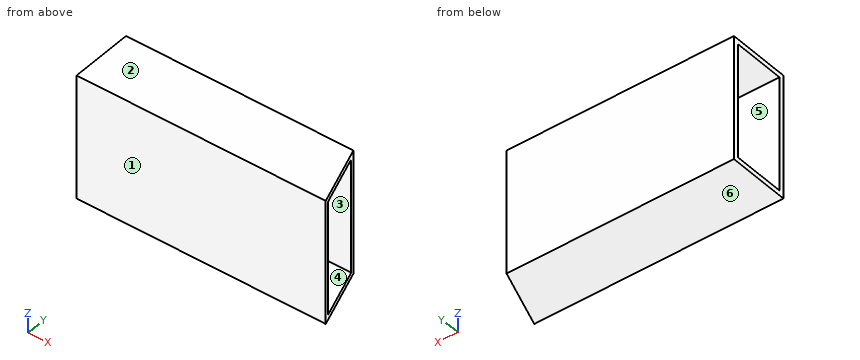
```python
from build123d import *

# Parameters (mm, degrees)
DODANIE_WYCI_GNI_CIE1_DEPTH = 100
SZKIC2_W                    = 92
SZKIC2_H                    = 42
WYTNIJ_WYCI_GNI_CIE1_DEPTH  = 200


with BuildPart() as part:
    # Szkic1 → Dodanie-wyciągnięcie1 (new body)
    with BuildSketch(Plane.XY):
        Polygon((0, 0), (200, 0), (182.5, 50), (0, 50), align=None)
    extrude(amount=DODANIE_WYCI_GNI_CIE1_DEPTH)

    # Szkic2 → Wytnij-wyciągnięcie1 (cut)
    with BuildSketch(Plane.ZY):
        with Locations((50, 25)):
            Rectangle(SZKIC2_W, SZKIC2_H)
    extrude(amount=-WYTNIJ_WYCI_GNI_CIE1_DEPTH, mode=Mode.SUBTRACT)


solid = part.part
```
Geometry: final body of the model. Coordinates: model frame, mm. Face numbers are marked on the shaded views. A direction names the side the tool comes from. Round coordinates to 2 decimals unless told otherwise and drop trailing zeros. Write each loop counter-clockwise with the first axis right and the second up, starting at its lowest first coordinate (ties: lowest second). Pieces come first, ordered by that corner, then holes.
Item 1: Material intervals for L1, parallel to Y at x = 166, z = 44; L2, parallel to Z at x = 19.5, y = 31.5; L3, parallel to X at y = 2.5, z = 72 (3 decimals), sorted ascending.
Item 2: Set-up query: the marked faces 5 and 6. Return all of +Z, -Z, +X, -X, +Y, -Y with unobstructed straight access to the full face (end or side cutting, diameter ignored); none if empty.
Item 3: Section query C-C (x = 137). Return loops of the section in (y, z), plus the area to 3 significant figures.
Item 4: Section query B-B (z = 74.5). Return loops of the section in (x, y).
Item 5: Mould query, pull axis Z, two halves, no side actions, for the marked faces 1, 2, 3 and 4. Classes: +Z half, -Z half, draft (parallel to the pull), parting line (faces both ways), or undercut.
Item 6: Section query A-A (y = 18). Return loops of the section in (x, z), plus the area to 3 significant figures.
Completed:
1. L1: y = 0 to 4, 46 to 50
1. L2: z = 0 to 4, 96 to 100
1. L3: x = 0 to 199.125
2. face 5: +X, -X
2. face 6: -Z, +X, -X, +Y, -Y
3. outline: (0, 0) - (50, 0) - (50, 100) - (0, 100) - close; hole (4, 4) - (46, 4) - (46, 96) - (4, 96) - close
3. area: 1,140 mm2
4. outline: (0, 0) - (200, 0) - (198.6, 4) - (0, 4) - close; (0, 46) - (183.9, 46) - (182.5, 50) - (0, 50) - close
5. face 1: draft
5. face 2: +Z half
5. face 3: undercut
5. face 4: undercut
6. outline: (0, 0) - (193.7, 0) - (193.7, 4) - (0, 4) - close; (0, 96) - (193.7, 96) - (193.7, 100) - (0, 100) - close
6. area: 1,550 mm2
